```python
from build123d import *

# Parameters (mm, degrees)
SKETCH1_W                = 29
SKETCH1_H                = 18
BOSS_EXTRUDE1_DEPTH      = 13
BOSS_EXTRUDE2_DEPTH      = 1.35
BOSS_EXTRUDE2_DEPTH_BACK = 14.35
CUT_EXTRUDE1_DEPTH       = 1.4
SHELL1_START             = -5.4
SHELL1_OUTLINE_W         = 24.6
SHELL1_OUTLINE_H         = 8.6
SHELL1_DEPTH             = 14.4
SHELL1_START_2           = -6.8
SHELL1_2_DEPTH           = 1.4
SKETCH4_R                = 1.05
CUT_EXTRUDE2_DEPTH       = 27.300807972
SKETCH5_W                = 2.257483773
SKETCH5_H                = 13
CUT_EXTRUDE3_DEPTH       = 0.5


# Read off the part's stored shape, not the designer's step: Shell1
with BuildPart() as part:
    # Sketch1 → Boss-Extrude1 (new body)
    with BuildSketch(Plane.XY):
        Rectangle(SKETCH1_W, SKETCH1_H)
    extrude(amount=BOSS_EXTRUDE1_DEPTH)

    # Sketch2 → Boss-Extrude2 (add, two sides: drawn at the far end of the back side and taken through both)
    with BuildSketch(Plane.XY.offset(13).offset(-BOSS_EXTRUDE2_DEPTH_BACK)):
        Polygon((-5.75, 1.8), (-5.25, 2.3), (5.25, 2.3), (5.75, 1.8), (8.25, 1.8), (8.25, 6.7), (-8.25, 6.7), (-8.25, 1.8), align=None)
    extrude(amount=BOSS_EXTRUDE2_DEPTH + BOSS_EXTRUDE2_DEPTH_BACK)

    # Sketch3 → Cut-Extrude1 (cut)
    with BuildSketch(Plane.XZ.offset(9)):
        with BuildLine():
            Line((-2.55, -6.5), (-2.55, 6.5))
            ThreePointArc((-2.55, 6.5), (0, 9.05), (2.55, 6.5))
            Line((2.55, 6.5), (2.55, -6.5))
            ThreePointArc((2.55, -6.5), (0, -9.05), (-2.55, -6.5))
        make_face()
        with BuildLine():
            Line((-21, 9.05), (-8, 9.05))
            ThreePointArc((-8, 9.05), (-5.45, 6.5), (-8, 3.95))
            Line((-8, 3.95), (-21, 3.95))
            ThreePointArc((-21, 3.95), (-23.55, 6.5), (-21, 9.05))
        make_face()
        with BuildLine():
            Line((21, 9.05), (8, 9.05))
            ThreePointArc((8, 9.05), (5.45, 6.5), (8, 3.95))
            Line((8, 3.95), (21, 3.95))
            ThreePointArc((21, 3.95), (23.55, 6.5), (21, 9.05))
        make_face()
    extrude(amount=-CUT_EXTRUDE1_DEPTH, mode=Mode.SUBTRACT)

    # Shell1 outline → Shell1 (cut)
    with BuildSketch(Plane(origin=(0, 0, 0), x_dir=(1, 0, 0), z_dir=(0, 1, 0)).offset(SHELL1_START)):
        with Locations((0, -6.5)):
            Rectangle(SHELL1_OUTLINE_W, SHELL1_OUTLINE_H)
    extrude(amount=SHELL1_DEPTH, mode=Mode.SUBTRACT)

    # Shell1 2 outline → Shell1 2 (cut)
    with BuildSketch(Plane(origin=(0, 0, 0), x_dir=(1, 0, 0), z_dir=(0, 1, 0)).offset(SHELL1_START_2)):
        with BuildLine():
            Line((2.018043607, -10.8), (5.981956393, -10.8))
            ThreePointArc((5.981956393, -10.8), (4.867971715, -10.071120108), (4, -9.061737691))
            ThreePointArc((4, -9.061737691), (3.132028285, -10.071120108), (2.018043607, -10.8))
        make_face()
        with BuildLine():
            ThreePointArc((4.75, -3.035898385), (5.333025611, -2.569383304), (5.981956393, -2.2))
            Line((5.981956393, -2.2), (4.75, -2.2))
            Line((4.75, -2.2), (4.75, -3.035898385))
        make_face()
        with BuildLine():
            Line((-5.981956393, -10.8), (-2.018043607, -10.8))
            ThreePointArc((-2.018043607, -10.8), (-3.132028285, -10.071120108), (-4, -9.061737691))
            ThreePointArc((-4, -9.061737691), (-4.867971715, -10.071120108), (-5.981956393, -10.8))
        make_face()
        with BuildLine():
            Line((-4.75, -3.035898385), (-4.75, -2.2))
            Line((-4.75, -2.2), (-5.981956393, -2.2))
            ThreePointArc((-5.981956393, -2.2), (-5.333025611, -2.569383304), (-4.75, -3.035898385))
        make_face()
    extrude(amount=SHELL1_2_DEPTH, mode=Mode.SUBTRACT)

    # Sketch4 → Cut-Extrude2 (cut, through all)
    with BuildSketch(Plane.XZ.offset(7.6)):
        with Locations((0, 6.5)):
            Circle(SKETCH4_R)
        with Locations((-8, 6.5)):
            Circle(SKETCH4_R)
        with Locations((8, 6.5)):
            Circle(SKETCH4_R)
    extrude(amount=-CUT_EXTRUDE2_DEPTH, mode=Mode.SUBTRACT)

    # Sketch5 → Cut-Extrude3 (cut)
    with BuildSketch(Plane(origin=(0, 9, 0), x_dir=(1, 0, 0), z_dir=(0, 1, 0))):
        with Locations((-13.371258114, -6.5)):
            Rectangle(SKETCH5_W, SKETCH5_H)
        with Locations((13.371258114, -6.5)):
            Rectangle(SKETCH5_W, SKETCH5_H)
    extrude(amount=-CUT_EXTRUDE3_DEPTH, mode=Mode.SUBTRACT)


solid = part.part
```
The listing builds one solid part. Answer for the finished solid, in the listing's coordinates (mm). A direction names the side the tool comes from. Coordinates: 2 decimals unless noted, no trailing zeros. Order: outer loops, then holes, each group sorted by start corner. A loop starts at its lowest first (then second) coordinate and runs counter-clockwise, first axis right, second up. Notation, with made-up numbers: M 74,53 L 112,53 A33 ccw 112,81 Z; hole C 22.25,-11 d2. An arc over 180 degrees is marked long. Answer as a JSON object with one key per item and string values. Group by question number.
1. Section C-C on x = -11 is taken. Write down the section's boundary in (y, z), then the cut area to 3 significant figures.
2. Straight lines are drawn through the part: line 1 (Z direction, x = 7.25, y = -1.5); line 2 (Z direction, x = 8, y = -5.85); line 3 (X direction, y = 7, z = 5). For each, find the intervals that lie inside material, in ascending order.
3. Section B-B on z = 0.75 is taken. Write down the section's boundary in (x, y).
4. Determine the mould class of faces 5 (the cylindrical face through (-4.9, -6.1, 10.1)), 6 (the flat face through (-13, 8.5, 6)), 7 (the cylindrical face through (-0.06, -8.31, 9.05)) for opening direction Z: released by +Z, released by -Z, zero draft, split by the parting line, or undercut.
5. Section D-D on y = 8 is taken. Write down the section's boundary in (x, z), then the cut area to 3 significant figures.
6. A tool of negligible diameter and unlimited length cuts with its end or side. For faces 1 (the flat face through (0, 6.7, 14)), 2 (the flat face through (2.55, -8, 3)), 3 (the flat face through (7, 1.8, 14)), 4 (the flat face through (0, -5.4, 5)), from which of +Z, -Z, +X, -X, +Y, -Y can it reach the whole face along a straight path? Write none if from no direction.
7. Section A-A on y = 5.75 is taken. Write down the section's boundary in (x, z).
8. Flat-ended cylindrical pins translate along their axes: P1, Ø5, axis at x = -5, z = 6.5, coming from the +Y side; P2, Ø1.5, axis at x = 12, y = -8.5, coming from the +Z side; P3, Ø8, axis at x = 0.5, y = -3, coming from the -Z side; P4, Ø1.9, axis at x = 0, z = 6.5, coming from the -Y side. Find the tip coordinate at first contact, or state that the pin passes through.
Values follow:
{
 "1": {"outline": "M -9,0 L 9,0 L 9,2.2 L -5.4,2.2 L -5.4,10.8 L 9,10.8 L 9,13 L -9,13 L -9,9.05 L -7.6,9.05 L -7.6,3.95 L -9,3.95 Z", "area": "103 mm2"},
 "2": {"line 1": "0 to 2.2, 10.8 to 13", "line 2": "0 to 5.45, 7.55 to 13", "line 3": "-14.5 to -12.3, 12.3 to 14.5"},
 "3": {"outline": "M -14.5,-9 L -2.55,-9 L -2.55,-7.6 L 2.55,-7.6 L 2.55,-9 L 14.5,-9 L 14.5,8.5 L 12.24,8.5 L 12.24,9 L -12.24,9 L -12.24,8.5 L -14.5,8.5 Z"},
 "4": {"face 5": "undercut", "face 6": "zero draft", "face 7": "released by -Z"},
 "5": {"outline": "M -14.5,0 L 14.5,0 L 14.5,13 L -14.5,13 Z; hole M -12.3,2.2 L 12.3,2.2 L 12.3,10.8 L -12.3,10.8 Z", "area": "165 mm2"},
 "6": {"face 1": "+Z, +X, -X, +Y", "face 2": "-Z, -Y", "face 3": "+Z, +X, -X, -Y", "face 4": "+Y"},
 "7": {"outline": "M -14.5,0 L -8.25,0 L -8.25,-1.35 L 8.25,-1.35 L 8.25,0 L 14.5,0 L 14.5,13 L 8.25,13 L 8.25,14.35 L -8.25,14.35 L -8.25,13 L -14.5,13 Z; hole M -12.3,2.2 L 12.3,2.2 L 12.3,10.8 L -12.3,10.8 Z"},
 "8": {"P1": "y = -5.4", "P2": "z = 13", "P3": "z = 0", "P4": "through"}
}
